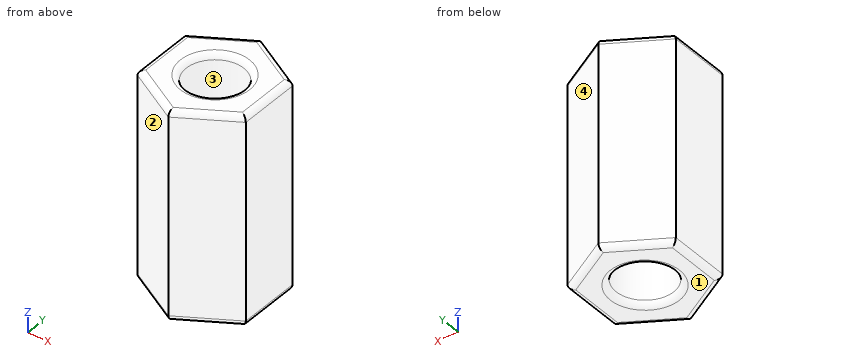
```python
from build123d import *

# Parameters (mm, degrees)
CROQUIS1_R              = 1.25
SALIENTE_EXTRUIR1_DEPTH = 9
REDONDEO1_R             = 0.25
REDONDEO2_R             = 0.25


with BuildPart() as part:
    # Croquis1 → Saliente-Extruir1 (new body)
    with BuildSketch(Plane.XY):
        Polygon((2.35, 1.356773133), (0, 2.713546265), (-2.35, 1.356773133), (-2.35, -1.356773133), (0, -2.713546265), (2.35, -1.356773133), align=None)
        Circle(CROQUIS1_R, mode=Mode.SUBTRACT)
    extrude(amount=SALIENTE_EXTRUIR1_DEPTH)

    # Redondeo1
    redondeo1_edges = [part.edges().sort_by_distance(p)[0] for p in [
        (-1.175, 2.035159699, 9),
        (-2.35, 0, 9),
        (-1.175, -2.035159699, 9),
        (1.175, -2.035159699, 9),
        (2.35, 0, 9),
        (1.175, -2.035159699, 0),
        (-1.175, -2.035159699, 0),
        (-2.35, 0, 0),
        (1.175, 2.035159699, 9),
        (-1.175, 2.035159699, 0),
        (1.175, 2.035159699, 0),
        (2.35, 0, 0),
    ]]
    fillet(redondeo1_edges, radius=REDONDEO1_R)

    # Redondeo2
    redondeo2_edges = [part.edges().sort_by_distance(p)[0] for p in [
        (-1.25, 0, 0),
        (-1.25, 0, 9),
    ]]
    fillet(redondeo2_edges, radius=REDONDEO2_R)


solid = part.part
```
Input: part model. Units: mm. Frame: model coordinates. Face numbers are marked on the shaded views. Give positions to 0.01 mm unless a question says otherwise; leave off trailing zeros. Order: outer loops, then holes, each group sorted by start corner. A loop starts at its lowest first (then second) coordinate and runs counter-clockwise, first axis right, second up.
1. Section B-B on y = 0. Return the cut outline in (x, z).
Derived:
outline: (-2.35, 0.25) arc R0.25 ccw to (-2.1, 0) - (-1.5, 0) arc R0.25 ccw to (-1.25, 0.25) - (-1.25, 8.75) arc R0.25 ccw to (-1.5, 9) - (-2.1, 9) arc R0.25 ccw to (-2.35, 8.75) - close; (1.25, 0.25) arc R0.25 ccw to (1.5, 0) - (2.1, 0) arc R0.25 ccw to (2.35, 0.25) - (2.35, 8.75) arc R0.25 ccw to (2.1, 9) - (1.5, 9) arc R0.25 ccw to (1.25, 8.75) - close
2. Pin query (flat end, axial travel): pin 1 (2 mm diameter, centred on x = 1.5, z = 1, fed in from +Y); pin 2 (2 mm diameter, centred on x = 1, y = 0, fed in from -Z); pin 3 (1.5 mm diameter, centred on x = 1.5, z = 1.5, fed in from +Y). Return the tip coordinate at first contact, or that it passes through.
Derived:
pin 1: stops at y = 2.42
pin 2: stops at z = 0
pin 3: stops at y = 2.28
3. Mould query, pull axis X, two halves, no side actions, for the marked faces 1, 2, 3 and 4. Classes: released by +X, released by -X, zero draft, split by the parting line, or undercut.
Derived:
face 1: zero draft
face 2: released by -X
face 3: undercut
face 4: released by +X
4. Material intervals for L1, parallel to Y at x = 0.45, z = 3; L2, parallel to Y at x = 2.1, z = 5.25; L3, parallel to X at y = 0.1, z = 7.5, sorted ascending.
Derived:
L1: y = -2.45 to -1.17, 1.17 to 2.45
L2: y = -1.5 to 1.5
L3: x = -2.35 to -1.25, 1.25 to 2.35
5. Section A-A on z = 4.5. Return the cut outline in (x, y), and give its area (3 significant figures).
Derived:
outline: (-2.35, -1.36) - (0, -2.71) - (2.35, -1.36) - (2.35, 1.36) - (0, 2.71) - (-2.35, 1.36) - close; hole circle Ø2.5 at (0, 0)
area: 14.2 mm2
